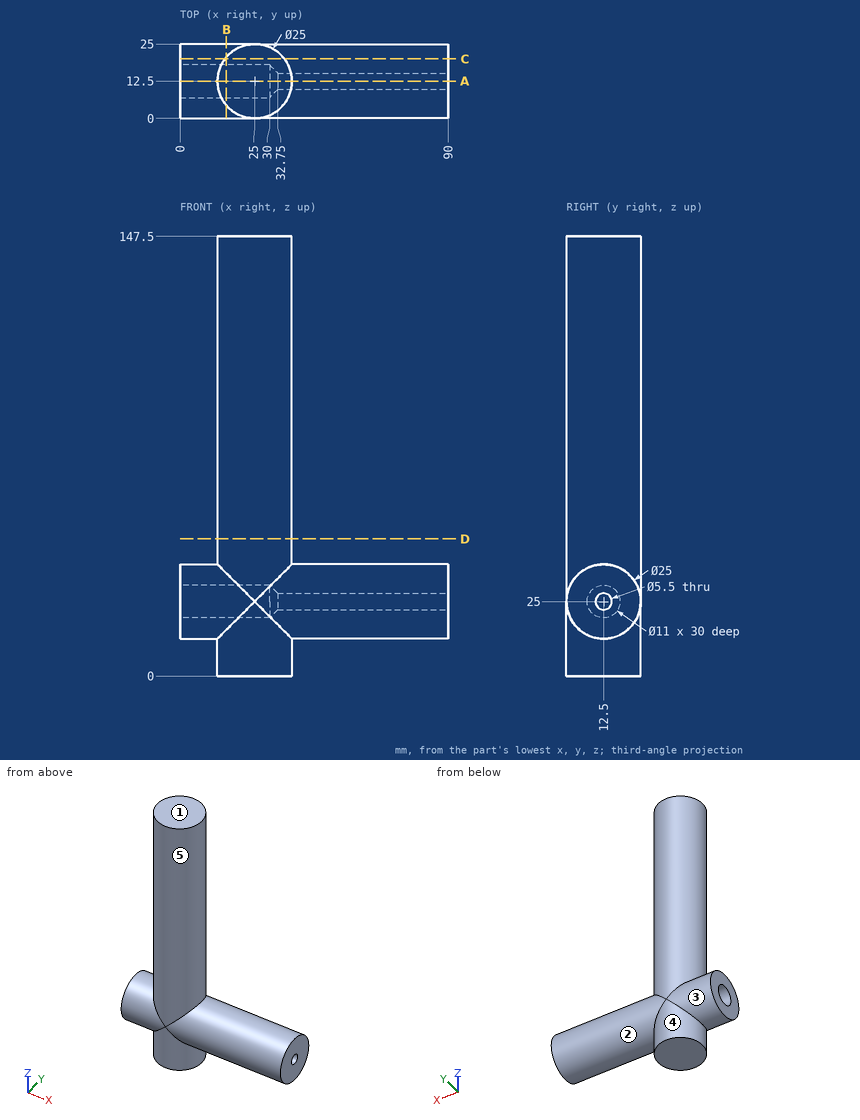
Source: three-view drawing plus pictorial views. Frame: mm from the lowest corner of the part. A direction names the side the tool comes from. Give positions to 0.01 mm unless a question says otherwise; leave off trailing zeros. Loops run counter-clockwise (first coordinate to the right, second up) from the corner with the lowest first, then second, coordinate; pieces in that order, holes last. Notation, with made-up numbers: (-5, 30) -> (13, 30) arc R17 cw to (13, 34) -> close; hole circle Ø7 at (38, 1). An arc over 180 degrees is marked (long way). Use a Markdown table: item, result. Add a question column.
(1) First-contact query: pin 1 Ø10 at (x, y) = (64, 3.5) entering from -Z; pin 2 Ø6 at (y, z) = (20, 132.5) entering from -X; pin 3 Ø5 at (x, z) = (66.5, 17.5) entering from -Y. Flat tips, straight axial feed; report the tip coordinate or a pass-through.
(2) Section query A-A (y = 12.5). Output: boundary loops of the cut face in (x, z).
(3) Section query B-B (x = 15.5). Output: boundary loops of the cut face in (y, z), then the cut area to 3 significant figures.
(4) Access query for the marked faces 1, 2, 3, 4 and 5. Directions: +Z, -Z, +X, -X, +Y, -Y. A direction counts if a zero-diameter tool reaches every point of the face in a straight line with its end or side. Return the directions, or none.
(5) Section query D-D (z = 46). Output: boundary loops of the cut face in (x, y).
(6) Section query C-C (y = 20). Output: boundary loops of the cut face in (x, z), then the cut area to 3 significant figures.
(7) Ray query, line 1 (Z direction, x = 9.25, y = 12.5); line 2 (Z direction, x = 73, y = 12.5); line 3 (X direction, y = 13, z = 68.5). Return the intervals inside material, ascending.
Checked values:
| question | item | result |
|---|---|---|
| 1 | pin 1 | z = 13.16 |
| 1 | pin 2 | x = 13.34 |
| 1 | pin 3 | y = 1.04 |
| 2 | outline | (0, 12.5) -> (12.5, 12.5) -> (12.5, 0) -> (37.5, 0) -> (37.5, 12.5) -> (90, 12.5) -> (90, 22.25) -> (32.75, 22.25) -> (30, 19.5) -> (0, 19.5) -> close; (0, 30.5) -> (30, 30.5) -> (32.75, 27.75) -> (90, 27.75) -> (90, 37.5) -> (37.5, 37.5) -> (37.5, 147.5) -> (12.5, 147.5) -> (12.5, 37.5) -> (0, 37.5) -> close |
| 3 | outline | (4.38, 0) -> (20.62, 0) -> (20.62, 15.5) arc R12.5 ccw to (20.62, 34.5) -> (20.62, 147.5) -> (4.38, 147.5) -> (4.38, 34.5) arc R12.5 ccw to (4.38, 15.5) -> close; hole circle Ø11 at (12.5, 25) |
| 3 | area | 2,420 mm^2 |
| 4 | face 1 | +Z, +X, -X, +Y, -Y |
| 4 | face 2 | +X |
| 4 | face 3 | -X |
| 4 | face 4 | -Z |
| 4 | face 5 | +Z |
| 5 | outline | circle Ø25 at (25, 12.5) |
| 6 | outline | (0, 15) -> (15, 15) -> (15, 0) -> (35, 0) -> (35, 15) -> (90, 15) -> (90, 35) -> (35, 35) -> (35, 147.5) -> (15, 147.5) -> (15, 35) -> (0, 35) -> close |
| 6 | area | 4,350 mm^2 |
| 7 | line 1 | 12.5 to 19.5, 30.5 to 37.5 |
| 7 | line 2 | 12.5 to 22.25, 27.75 to 37.5 |
| 7 | line 3 | 12.51 to 37.49 |
